Here's how the part is built. I have some questions about the finished solid (model axes, mm). A direction names the side the tool comes from. Coordinates: 2 decimals unless noted, no trailing zeros. Loops run counter-clockwise (first coordinate to the right, second up) from the corner with the lowest first, then second, coordinate; pieces in that order, holes last. Notation, with made-up numbers: (70.25, 61) - (80.25, 61) arc R10 ccw to (80.25, 78) - close; hole circle Ø3 at (9, 74.5). An arc over 180 degrees is marked (long way). Use a Markdown table: item, result.
Autodesk Inventor part; units mm, degrees
ref_plane "YZ Plane" through (0, 0, 0) normal (1, 0, 0) x (0, 1, 0)
ref_plane "XZ Plane" through (0, 0, 0) normal (0, 1, 0) x (-1, 0, 0)
ref_plane "XY Plane" through (0, 0, 0) normal (0, 0, 1) x (1, 0, 0)
sketch "Sketch1" plane through (0, 0, 0) normal (1, 0, 0) x (0, 1, 0)
  line L0 (-7.5231, -44.0814) -> (7.8367, -44.0814)
  line L1 (7.8367, -44.0814) -> (7.8367, 45.9186)
  line L2 (7.8367, 45.9186) -> (-8.1633, 45.9186)
  line L3 (-7.5231, -44.0814) -> (7.8367, 45.9186) construction
  line L4 (7.8367, -44.0814) -> (-8.1633, 45.9186) construction
  line L5 (-8.1633, 45.9186) -> (-8.1633, -15.5814)
  line L6 (3.8367, -15.5814) -> (-8.1633, -15.5814)
  line L7 (3.8367, -15.5814) -> (3.8367, -39.0814)
  line L8 (3.8367, -39.0814) -> (-7.5231, -39.0814)
  line L9 (-7.5231, -39.0814) -> (-7.5231, -44.0814)
  point P0 (0, 0)
  dimension "d0" = 16
  dimension "d1" = 90
  dimension "d24" = 12
  dimension "d28" = 5
  dimension "d29" = 23.5
extrude "Extrusion1" add sketch "Sketch1" along normal blind 6
sketch "Sketch2" plane through (6, 0, 0) normal (1, 0, 0) x (0, 0, -1)
  point P0 (0, 0)
sketch "Sketch3" plane through (6, 0, 0) normal (1, 0, 0) x (0, 0, -1)
  line L0 (-45.9186, 7.8367) -> (-45.9186, -8.1633)
  line L1 (44.0814, -7.5231) -> (44.0814, 7.8367)
  point P0 (0, 0)
  point P1 (-34.9186, -0.1633)
  point P2 (27.0814, 0.4769)
  point P3 (-42.4186, -0.1633)
  dimension "d4" = 11
  dimension "d5" = 17
  dimension "d23" = 7.5
hole "Hole1" at (6, -0.1633, 34.9186) at (6, -0.1633, 42.4186) direction (-1, 0, 0) diameter 2.5 end through all
fillet "Fillet1" radius 2 4 edges at (3, 7.8367, 45.9186) (3, -8.1633, 45.9186) (3, 7.8367, -44.0814) (3, -7.5231, -44.0814)
sketch "Sketch4" plane through (6, 0, 0) normal (1, 0, 0) x (0, 0, -1)
  line L0 (44.0814, -5.5231) -> (44.0814, 5.8367)
  line L1 (-43.9186, -8.1633) -> (15.5814, -8.1633)
  line L2 (39.0814, -7.5231) -> (42.0814, -7.5231)
  point P0 (0, 0)
  point P1 (41.5814, -1.5231)
  point P2 (12.8885, -2.1633)
  dimension "d14" = 2.5
  dimension "d15" = 28.7
  dimension "d30" = 6
  dimension "d31" = 6
hole "Hole2" at (6, -2.1633, -12.8885) at (6, -1.5231, -41.5814) direction (-1, 0, 0) diameter 2 end through all
properties part number "Arm1"
Q1. I want a section at B-B, the plane z = -26.5. Write out the boundary of the cut face in (x, y).
Check values:
| item | result |
|---|---|
| outline | (0, 3.84) - (6, 3.84) - (6, 7.84) - (0, 7.84) - close |
Q2. Will these pins go through, and if not, where does the flat tip stop? P1, Ø3, axis at y = -0.16, z = 34.92, coming from the +X side; P2, Ø3.5, axis at x = 2, z = -41, coming from the -Y side; P3, Ø1.8, axis at x = 2.5, z = -27.5, coming from the -Y side.
Check values:
| item | result |
|---|---|
| P1 | x = 6 |
| P2 | y = -7.52 |
| P3 | y = 3.84 |
Q3. Which directions (+Z, -Z, +X, -X, +Y, -Y) give clear straight access to the entire face, cutting with the end or side of a thin tool? Please do faces 5 (the face through (3, 0, -44.081)), 6 (the face through (3, -7.523, -41)), 7 (the face through (3, -2, -39.081)).
Check values:
| item | result |
|---|---|
| face 5 | -Z, +X, -X, +Y, -Y |
| face 6 | -Z, +X, -X, -Y |
| face 7 | +X, -X, -Y |
Q4. I want a section at A-A, the plane x = 4.5. Write out the boundary of the cut face in (y, z).
Check values:
| item | result |
|---|---|
| outline | (-8.16, -15.58) - (3.84, -15.58) - (3.84, -39.08) - (-7.52, -39.08) - (-7.52, -42.08) arc R2 ccw to (-5.52, -44.08) - (5.84, -44.08) arc R2 ccw to (7.84, -42.08) - (7.84, 43.92) arc R2 ccw to (5.84, 45.92) - (-6.16, 45.92) arc R2 ccw to (-8.16, 43.92) - close; hole circle Ø2 at (-2.16, -12.89); hole circle Ø2 at (-1.52, -41.58); hole circle Ø2.5 at (-0.16, 34.92); hole circle Ø2.5 at (-0.16, 42.42) |
Q5. If we mould it in two halves opening along Z, with no side actions, what happens to faces 1 (the face through (3, -8.163, 15)), 2 (the face through (2.958, -1.823, -42.535)), 3 (the face through (2.958, -0.539, 33.726)), 4 (the face through (3.042, 7.266, 45.317))? For each: pulls with the +Z half, pulls with the -Z half, needs draft (parallel to the pull), parting line crosses it, or undercut.
Check values:
| item | result |
|---|---|
| face 1 | needs draft |
| face 2 | undercut |
| face 3 | undercut |
| face 4 | pulls with the +Z half |
Q6. Please list where these lines run through material, in increasing order: L1, parallel to Z at x = 3.6, y = -0.25; L2, parallel to Z at x = 3, y = -2.75; L3, parallel to Z at x = 4.1, y = -2. Write a range as from..to.
Check values:
| item | result |
|---|---|
| L1 | -44.08..-39.08, -15.58..33.67, 36.17..41.17, 43.67..45.92 |
| L2 | -44.08..-39.08, -15.58..-13.7, -12.08..45.92 |
| L3 | -44.08..-42.46, -40.7..-39.08, -15.58..-13.88, -11.9..45.92 |
